Geometry check sheet. Reference: the model listing, model coordinates, mm. A direction names the side the tool comes from. Coordinates: 2 decimals unless noted, no trailing zeros. Write each loop counter-clockwise with the first axis right and the second up, starting at its lowest first coordinate (ties: lowest second). Pieces come first, ordered by that corner, then holes. Notation, with made-up numbers: (-32, 9) -> (-10, 9) arc R20 ccw to (-10, 22) -> close; hole circle Ø10 at (-33.75, -39). An arc over 180 degrees is marked (long way). Put each result on its own line as item: value. Start each with the question number.
from build123d import *

# Parameters (mm, degrees)
SKETCH_1_R          = 12.5
EXTRUDE_1_DEPTH     = 29
CUT_EXTRUDE_START   = -1.5
SKETCH_2_R          = 12.5
SKETCH_2_R_2        = 11
CUT_EXTRUDE_1_DEPTH = 1.5
FILLET_1_R          = 0.5
SKETCH_3_R          = 6
EXTRUDE_2_DEPTH     = 2
SKETCH_4_R          = 2
EXTRUDE_3_DEPTH     = 10
CUT_EXTRUDE_START_2 = -8
CUT_EXTRUDE_2_DEPTH = 8
SKETCH_6_R          = 4
EXTRUDE_4_DEPTH     = 5.5
SKETCH_7_R          = 1.75
EXTRUDE_5_DEPTH     = 10
SKETCH_8_R          = 1.5
CUT_EXTRUDE_3_DEPTH = 4


with BuildPart() as part:
    # ｽｹｯﾁ1 → ﾎﾞｽ - 押し出し1 (new body)
    with BuildSketch(Plane(origin=(0, 0, 0), x_dir=(0, 0, -1), z_dir=(1, 0, 0))):
        with Locations(Location((0, 0, 0), (0, 0, 180))):
            Circle(SKETCH_1_R)
    extrude(amount=EXTRUDE_1_DEPTH)

    # ｽｹｯﾁ2 → ｶｯﾄ - 押し出し1 (cut)
    with BuildSketch(Plane(origin=(27, 0, 0), x_dir=(0, 0, -1), z_dir=(1, 0, 0)).offset(CUT_EXTRUDE_START)):
        with Locations(Location((0, 0, 0), (0, 0, 180))):
            Circle(SKETCH_2_R)
        Circle(SKETCH_2_R_2, mode=Mode.SUBTRACT)
    extrude(amount=CUT_EXTRUDE_1_DEPTH, mode=Mode.SUBTRACT)

    # ﾌｨﾚｯﾄ1
    fillet_1_edges = [part.edges().sort_by_distance(p)[0] for p in [
        (0, 0, -12.5),
        (29, 0, -12.5),
    ]]
    fillet(fillet_1_edges, radius=FILLET_1_R)

    # ｽｹｯﾁ3 → ﾎﾞｽ - 押し出し2 (add)
    with BuildSketch(Plane(origin=(29, 0, 0), x_dir=(0, 0, -1), z_dir=(1, 0, 0))):
        Circle(SKETCH_3_R)
    extrude(amount=EXTRUDE_2_DEPTH)

    # ｽｹｯﾁ4 → ﾎﾞｽ - 押し出し3 (add)
    with BuildSketch(Plane(origin=(31, 0, 0), x_dir=(0, 0, -1), z_dir=(1, 0, 0))):
        Circle(SKETCH_4_R)
    extrude(amount=EXTRUDE_3_DEPTH)

    # ｽｹｯﾁ5 → ｶｯﾄ - 押し出し2 (cut)
    with BuildSketch(Plane(origin=(41, 0, 0), x_dir=(0, 0, -1), z_dir=(1, 0, 0)).offset(CUT_EXTRUDE_START_2)):
        with BuildLine():
            Line((-1.2, 1.6), (1.2, 1.6))
            ThreePointArc((1.2, 1.6), (0, 2), (-1.2, 1.6))
        make_face()
    extrude(amount=CUT_EXTRUDE_2_DEPTH, mode=Mode.SUBTRACT)

    # ｽｹｯﾁ6 → ﾎﾞｽ - 押し出し4 (add)
    with BuildSketch(Plane.ZY):
        with Locations(Location((0, -6, 0), (0, 0, 180))):
            Circle(SKETCH_6_R)
    extrude(amount=EXTRUDE_4_DEPTH)

    # ｽｹｯﾁ7 → ﾎﾞｽ - 押し出し5 (add)
    with BuildSketch(Plane.ZY.offset(5.5)):
        with Locations((0, -6)):
            Circle(SKETCH_7_R)
    extrude(amount=EXTRUDE_5_DEPTH)

    # ｽｹｯﾁ8 → ｶｯﾄ - 押し出し3 (cut)
    with BuildSketch(Plane(origin=(29, 0, 0), x_dir=(0, 0, -1), z_dir=(1, 0, 0))):
        with Locations((-9, 0)):
            Circle(SKETCH_8_R)
        with Locations(Location((9, 0, 0), (0, 0, 180))):
            Circle(SKETCH_8_R)
    extrude(amount=-CUT_EXTRUDE_3_DEPTH, mode=Mode.SUBTRACT)


solid = part.part
Item 1: Section check D-D, the plane x = 21. Enter the section's corners in (y, z).
Item 2: Scan lines: line 1 along X through (y, z) = (-9.25, -7.5); line 2 along X through (y, z) = (2, 5.5); line 3 along X through (y, z) = (3, 9). Record each from-to range of solid material in increasing order. Write a range as [from, to].
Item 3: Access from +Z, -Z, +X, -X, +Y, -Y to the whole of each face (thin tool, end or side, straight path). Record for faces 5 (the flat face through (27, 10, 5)), 6 (the flat face through (31, 0, -3)), 7 (the flat face through (-5.5, -4, -1)).
Item 4: Go/stop test with flat-tipped pins: P1, Ø10, axis at x = 22.5, z = 10, coming from the -Y side; P2, Ø2, axis at x = 26.5, z = -4, coming from the -Y side; P3, Ø7.5, axis at y = 4, z = -5, coming from the -X side. Record where each tip stops, or that it passes through.
Item 5: Mould release check, pull along X, two halves, no side actions. Record for faces 1 (the cylindrical face through (26.24, -10.74, 2.38)), 2 (the flat face through (37, 1.6, 0)), 3 (the flat face through (29, 2, -6)), 4 (the flat face through (0, 0, 0)): released by +X, released by -X, zero draft, split by the parting line, or undercut.
Item 6: Section check C-C, the plane x = 30. Enter the section's corners in (y, z), and give its area (3 significant figures).
From the geometry:
1. outline: circle Ø25 at (0, 0)
2. line 1: [0, 25.5], [27, 29]
2. line 2: [0, 31]
2. line 3: [0, 29]
3. face 5: none
3. face 6: +X
3. face 7: -X
4. P1: y = -11.46
4. P2: y = -12.1
4. P3: x = 0
5. face 1: undercut
5. face 2: zero draft
5. face 3: released by +X
5. face 4: released by -X
6. outline: circle Ø12 at (0, 0)
6. area: 113 mm²
